Read the model definition and answer for the solid it produces. Units are mm, in the model's axes. A direction names the side the tool comes from. Round coordinates to 2 decimals unless told otherwise and drop trailing zeros. Order: outer loops, then holes, each group sorted by start corner. A loop starts at its lowest first (then second) coordinate and runs counter-clockwise, first axis right, second up. Notation, with made-up numbers: (34, -31.5) - (60, -31.5) arc R13 cw to (60, -9.5) - close; hole circle Ø8 at (87, 70). An arc over 180 degrees is marked (long way). Put each result on its own line as item: value. Start each with the question number.
Q1. Find the intervals of material crossed by line 1 along X through (y, z) = (-0.75, -8.5); line 2 along Z through (x, y) = (5, 1.75); line 3 along Y through (x, z) = (0, -2.5), in increasing order. Write a range as from..to.
Q2. Section D-D on y = -5.5 is taken. Give the vertices of the cut face in (x, z).
Q3. Which of the six approach directions +Z, -Z, +X, -X, +Y, -Y give full straight-line access (tool end or side, diameter ignored) to faces 4 (the face through (-3, 0, 0)), 5 (the face through (-2.5, 0, 0)), 6 (the face through (-4, 0, 10))?
Q4. Each of these flat-tipped pins is pushed along its axis until it touches: pin 1 Ø1.5 at (x, z) = (-0.5, 5.5) entering from -Y; pin 2 Ø1.5 at (x, z) = (0.5, -5.5) entering from +Y; pin 3 Ø5.5 at (y, z) = (-0.5, -1) entering from -X. Where does it stop, or does it pass through?
Q5. Section B-B on z = 1.5 is taken. Give the vertices of the cut face in (x, y).
Q6. Section A-A on x = 0 is taken. Give the vertices of the cut face in (y, z), then the cut area to 3 significant figures.
Q7. Section C-C on y = -1 is taken. Give the vertices of the cut face in (x, z).
Q8. For a pull along Y with two mould halves and no side action, classify faces 1 (the face through (0, -3, 0)), 2 (the face through (2, 7, 11)), 3 (the face through (-2, -7, -11)) as pulls with the +Y half, pulls with the -Y half, needs draft (parallel to the pull), parting line crosses it, or undercut.
from build123d import *

# Parameters (mm, degrees)
SKETCH_1_W               = 6
SKETCH_1_H               = 7
SKETCH_1_W_2             = 5
SKETCH_1_H_2             = 6
EXTRUDE_1_DEPTH          = 11.5
SKETCH_2_W               = 6
SKETCH_2_H               = 7
EXTRUDE_2_DEPTH          = 1.5
SKETCH_3_R               = 19.100398606
SKETCH_3_W               = 18.715870292
SKETCH_3_H               = 14
CUT_EXTRUDE_1_DEPTH      = 26.719642299
CUT_EXTRUDE_2_DEPTH      = 25.904818811
CUT_EXTRUDE_3_DEPTH      = 25.904818811
CUT_EXTRUDE_3_DEPTH_BACK = 25.904818811
FILLET_1_R               = 0.2


with BuildPart() as part:
    # 草图1 → 凸台-拉伸1 (new, symmetric)
    with BuildSketch(Plane.XY):
        Rectangle(SKETCH_1_W, SKETCH_1_H)
        Rectangle(SKETCH_1_W_2, SKETCH_1_H_2, mode=Mode.SUBTRACT)
    extrude(amount=EXTRUDE_1_DEPTH, both=True)

    # 草图2 → 凸台-拉伸2 (add)
    with BuildSketch(Plane.XY.offset(11.5)):
        with BuildLine():
            Line((-6.5, 6.92820323), (-6.5, -6.92820323))
            ThreePointArc((-6.5, -6.92820323), (0, -9.5), (6.5, -6.92820323))
            Line((6.5, -6.92820323), (6.5, 6.92820323))
            ThreePointArc((6.5, 6.92820323), (0, 9.5), (-6.5, 6.92820323))
        make_face()
        Rectangle(SKETCH_2_W, SKETCH_2_H, mode=Mode.SUBTRACT)
    extrude_2 = extrude(amount=-EXTRUDE_2_DEPTH)

    # 镜向1: 凸台-拉伸2 across plane
    add(extrude_2.mirror(Plane.XY))

    # 草图3 → 切除-拉伸1 (cut, through all)
    with BuildSketch(Plane.XY.offset(11.5)):
        Circle(SKETCH_3_R)
        Rectangle(SKETCH_3_W, SKETCH_3_H, mode=Mode.SUBTRACT)
    extrude(amount=-CUT_EXTRUDE_1_DEPTH, mode=Mode.SUBTRACT)

    # 草图4 → 切除-拉伸2 (cut, through all)
    with BuildSketch(Plane.XY.offset(11.5)):
        with BuildLine():
            Line((-6.5, 6.92820323), (-6.5, 3))
            ThreePointArc((-6.5, 3), (-5.328427125, 5.828427125), (-2.5, 7))
            Line((-2.5, 7), (-6.422616289, 7))
            ThreePointArc((-6.422616289, 7), (-6.461407868, 6.964209098), (-6.5, 6.92820323))
        make_face()
        with BuildLine():
            ThreePointArc((2.5, 7), (5.328427125, 5.828427125), (6.5, 3))
            Line((6.5, 3), (6.5, 6.92820323))
            ThreePointArc((6.5, 6.92820323), (6.461407868, 6.964209098), (6.422616289, 7))
            Line((6.422616289, 7), (2.5, 7))
        make_face()
        with BuildLine():
            ThreePointArc((6.5, -3), (5.328427127, -5.828427123), (2.500000005, -7))
            Line((2.500000005, -7), (6.422616289, -7))
            ThreePointArc((6.422616289, -7), (6.461407868, -6.964209098), (6.5, -6.92820323))
            Line((6.5, -6.92820323), (6.5, -3))
        make_face()
        with BuildLine():
            ThreePointArc((-6.5, -6.92820323), (-6.461407868, -6.964209098), (-6.422616289, -7))
            Line((-6.422616289, -7), (-2.499999995, -7))
            ThreePointArc((-2.499999995, -7), (-5.328427123, -5.828427127), (-6.5, -3))
            Line((-6.5, -3), (-6.5, -6.92820323))
        make_face()
    extrude(amount=-CUT_EXTRUDE_2_DEPTH, mode=Mode.SUBTRACT)

    # 草图5 → 切除-拉伸3 (cut, two sides: drawn at the far end of the back side and taken through both)
    with BuildSketch(Plane.XY.offset(11.5).offset(-CUT_EXTRUDE_3_DEPTH_BACK)):
        with BuildLine():
            Line((1, 6.25), (1, 7))
            Line((1, 7), (-1, 7))
            Line((-1, 7), (-1, 6.25))
            ThreePointArc((-1, 6.25), (0, 5.25), (1, 6.25))
        make_face()
        with BuildLine():
            Line((1, -7), (1, -6.25))
            ThreePointArc((1, -6.25), (0, -5.25), (-1, -6.25))
            Line((-1, -6.25), (-1, -7))
            Line((-1, -7), (1, -7))
        make_face()
    extrude(amount=CUT_EXTRUDE_3_DEPTH + CUT_EXTRUDE_3_DEPTH_BACK, mode=Mode.SUBTRACT)

    # 圆角1
    fillet_1_edges = [part.edges().sort_by_distance(p)[0] for p in [
        (-3, 3.5, 0),
        (3, 3.5, 0),
        (3, -3.5, 0),
        (-3, -3.5, 0),
    ]]
    fillet(fillet_1_edges, radius=FILLET_1_R)


solid = part.part
Findings:
1. line 1: -3..-2.5, 2.5..3
1. line 2: -11.5..-10, 10..11.5
1. line 3: -3.5..-3, 3..3.5
2. outline: (-5.62, -11.5) - (-0.66, -11.5) - (-0.66, -10) - (-5.62, -10) - close; (-5.62, 10) - (-0.66, 10) - (-0.66, 11.5) - (-5.62, 11.5) - close; (0.66, -11.5) - (5.62, -11.5) - (5.62, -10) - (0.66, -10) - close; (0.66, 10) - (5.62, 10) - (5.62, 11.5) - (0.66, 11.5) - close
3. face 4: -X, +Y, -Y
3. face 5: +Z, -Z
3. face 6: none
4. pin 1: y = -3.5
4. pin 2: y = 3.5
4. pin 3: x = -3
5. outline: (-3, -3.3) arc R0.2 ccw to (-2.8, -3.5) - (2.8, -3.5) arc R0.2 ccw to (3, -3.3) - (3, 3.3) arc R0.2 ccw to (2.8, 3.5) - (-2.8, 3.5) arc R0.2 ccw to (-3, 3.3) - close; hole (-2.5, -3) - (2.5, -3) - (2.5, 3) - (-2.5, 3) - close
6. outline: (-5.25, -11.5) - (-3, -11.5) - (-3, 11.5) - (-5.25, 11.5) - (-5.25, 10) - (-3.5, 10) - (-3.5, -10) - (-5.25, -10) - close; (3, -11.5) - (5.25, -11.5) - (5.25, -10) - (3.5, -10) - (3.5, 10) - (5.25, 10) - (5.25, 11.5) - (3, 11.5) - close
6. area: 33.5 mm2
7. outline: (-6.5, -11.5) - (-2.5, -11.5) - (-2.5, 11.5) - (-6.5, 11.5) - (-6.5, 10) - (-3, 10) - (-3, -10) - (-6.5, -10) - close; (2.5, -11.5) - (6.5, -11.5) - (6.5, -10) - (3, -10) - (3, 10) - (6.5, 10) - (6.5, 11.5) - (2.5, 11.5) - close
8. face 1: undercut
8. face 2: pulls with the +Y half
8. face 3: pulls with the -Y half
